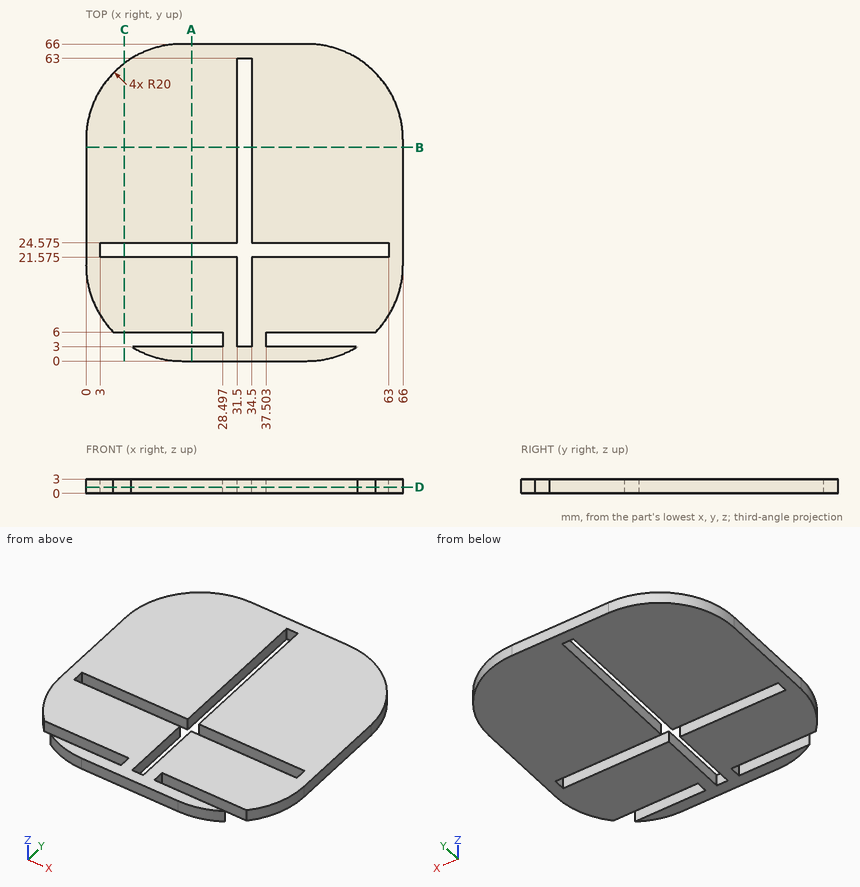
Design review of the part shown in the three views and the two pictorial views. Dimensions are in mm from the part's minimum x, y and z. Coordinates: 2 decimals unless noted, no trailing zeros. Loops run counter-clockwise (first coordinate to the right, second up) from the corner with the lowest first, then second, coordinate; pieces in that order, holes last.
Q1. For pin 1 (0.9 mm diameter, centred on x = 12, z = 2, fed in from -Y); pin 2 (1.5 mm diameter, centred on x = 53.5, z = 1, fed in from +Y); pin 3 (0.9 mm diameter, centred on y = 47.5, z = 2, fed in from +X), all flat-tipped, find the tip position at first contact; note any pin that passes through.
Reported:
pin 1: stops at y = 1.48
pin 2: stops at y = 64.83
pin 3: stops at x = 65.97
Q2. To check wall thickness, follow line 1 (Y direction, x = 44, z = 1.05) (3 decimals); line 2 (X direction, y = 34.5, z = 2.2); line 3 (Y direction, x = 31, z = 1.55) (3 decimals). State the ranges of each line that lie inside material, in increasing order.
Reported:
line 1: y = 0 to 3, 6 to 21.575, 24.575 to 66
line 2: x = 0 to 31.5, 34.5 to 66
line 3: y = 0 to 21.575, 24.575 to 66
Q3. We need section D-D on z = 1.3. State the section outline as (x, y) points (1 decimal), and give its area (3 significant figures).
Reported:
outline: (0, 20) arc R20 ccw to (5.7, 6) - (28.5, 6) - (28.5, 3) - (9.5, 3) arc R20 ccw to (20, 0) - (46, 0) arc R20 ccw to (56.5, 3) - (37.5, 3) - (37.5, 6) - (60.3, 6) arc R20 ccw to (66, 20) - (66, 46) arc R20 ccw to (46, 66) - (20, 66) arc R20 ccw to (0, 46) - close; hole (3, 21.6) - (31.5, 21.6) - (31.5, 3) - (34.5, 3) - (34.5, 21.6) - (63, 21.6) - (63, 24.6) - (34.5, 24.6) - (34.5, 63) - (31.5, 63) - (31.5, 24.6) - (3, 24.6) - close
area: 3,540 mm2
Q4. We need section C-C on x = 8. State the section outline as (y, z) points (3 decimals).
Reported:
outline: (6, 0) - (21.575, 0) - (21.575, 3) - (6, 3) - close; (24.575, 0) - (62, 0) - (62, 3) - (24.575, 3) - close
Q5. We need section B-B on y = 44.5. State the section outline as (x, z) points, and give its area (3 significant figures).
Reported:
outline: (0, 0) - (31.5, 0) - (31.5, 3) - (0, 3) - close; (34.5, 0) - (66, 0) - (66, 3) - (34.5, 3) - close
area: 189 mm2
Q6. We need section A-A on x = 22. State the section outline as (y, z) points (3 decimals).
Reported:
outline: (0, 0) - (3, 0) - (3, 3) - (0, 3) - close; (6, 0) - (21.575, 0) - (21.575, 3) - (6, 3) - close; (24.575, 0) - (66, 0) - (66, 3) - (24.575, 3) - close
